```python
from build123d import *


with BuildPart() as f1:
    # F0 (on Front) → F1 (revolve)
    with BuildSketch(Plane.XZ):
        with BuildLine():
            Line((-6.856, 5), (-8, 5))
            Line((-8, 5), (-8, 0))
            Line((-8, 0), (-6.856, 0))
            Line((-6.856, 0), (-6.856, 1.43))
            ThreePointArc((-6.856, 1.43), (-6, 1.1297314132), (-5.144, 1.43))
            Line((-5.144, 1.43), (-5.144, 0))
            Line((-5.144, 0), (-4, 0))
            Line((-4, 0), (-4, 5))
            Line((-4, 5), (-5.144, 5))
            Line((-5.144, 5), (-5.144, 3.57))
            ThreePointArc((-5.144, 3.57), (-6, 3.8702685868), (-6.856, 3.57))
            Line((-6.856, 3.57), (-6.856, 5))
        make_face()
    revolve(axis=Axis((0, 0, 1.894922927), (0, 0, -1)))


solid = f1.part
```
Check sheet for the modelled part. Datum: model origin and axes. Units: mm. A direction names the side the tool comes from. Coordinates: 2 decimals unless noted, no trailing zeros. Write each loop counter-clockwise with the first axis right and the second up, starting at its lowest first coordinate (ties: lowest second). Pieces come first, ordered by that corner, then holes. Notation, with made-up numbers: M 49,60.25 L 103,60.25 A27 cw 103,90.25 Z; hole C 76.5,-25.5 d6. An arc over 180 degrees is marked long. Write item = value, one per line. Start each with the question number.
1. Tool access check on faces 4 (the cylindrical face through (-4.906, 1.545, 0.705)), 5 (the flat face through (6, 4, 5)), 6 (the cylindrical face through (5.44, -4.17, 4.3)). Record the directions out of +Z, -Z, +X, -X, +Y, -Y that give a thin tool (end or side, any length) a straight path to the whole face; none if there is none.
2. Mould release check, pull along Y, two halves, no side actions. Record for faces 1 (the cylindrical face through (5.44, -4.17, 0.73)), 2 (the flat face through (3, -3, 5)), 3 (the cylindrical face through (1.73, -7.81, 2.46)): pulls with the +Y half, pulls with the -Y half, needs draft (parallel to the pull), parting line crosses it, or undercut.
3. Thickness scan on probe 1 along Y at (x, z) = (0, 4.05); probe 2 along Y at (x, z) = (-3, 0.6); probe 3 along X at (y, z) = (4.25, 0.55). Record the ranges inside material, lowest first.
4. Go/stop test with a flat-tipped pin: pin 1 (1.5 mm diameter, centred on y = 5, z = 1, fed in from -X). Record where the tip stops, or that it passes through.
5. Sectioned sample at A-A (x = 0). Record the cut outline in (y, z).
6. Sectioned sample at C-C (z = 4.7). Record the cut outline in (x, y).
The answers:
q1.face_4 = -Z
q1.face_5 = +Z, +X, -X, +Y, -Y
q1.face_6 = +Z
q2.face_1 = undercut
q2.face_2 = needs draft
q2.face_3 = parting line crosses it
q3.probe_1 = -8 to -6.86, -5.14 to -4, 4 to 5.14, 6.86 to 8
q3.probe_2 = -7.42 to -6.16, -4.18 to -2.65, 2.65 to 4.18, 6.16 to 7.42
q3.probe_3 = -6.78 to -5.38, -2.9 to 2.9, 5.38 to 6.78
q4.pin_1 = -6.78
q5.outline = M -8,0 L -6.86,0 L -6.86,1.43 A1.37 ccw -5.14,1.43 L -5.14,0 L -4,0 L -4,5 L -5.14,5 L -5.14,3.57 A1.37 ccw -6.86,3.57 L -6.86,5 L -8,5 Z; M 4,0 L 5.14,0 L 5.14,1.43 A1.37 ccw 6.86,1.43 L 6.86,0 L 8,0 L 8,5 L 6.86,5 L 6.86,3.57 A1.37 ccw 5.14,3.57 L 5.14,5 L 4,5 Z
q6.outline = C 0,0 d16; C 0,0 d10.29; hole C 0,0 d13.71; hole C 0,0 d8
